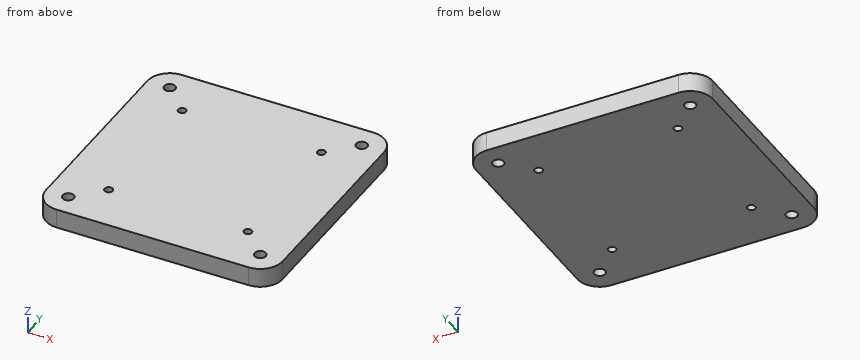
```python
from build123d import *

# Parameters (mm, degrees)
ESQUISSE1_W        = 74
ESQUISSE1_H        = 74
ESQUISSE1_R        = 1.75
ESQUISSE1_R_2      = 1.25
BOSS_EXTRU_1_DEPTH = 6
CONG_1_R           = 7


with BuildPart() as part:
    # Esquisse1 → Boss.-Extru.1 (new body)
    with BuildSketch(Plane.XY):
        Rectangle(ESQUISSE1_W, ESQUISSE1_H)
        with Locations((-30, 30)):
            Circle(ESQUISSE1_R, mode=Mode.SUBTRACT)
        with Locations((-21.75, 21.75)):
            Circle(ESQUISSE1_R_2, mode=Mode.SUBTRACT)
        with Locations((30, 30)):
            Circle(ESQUISSE1_R, mode=Mode.SUBTRACT)
        with Locations((21.75, 21.75)):
            Circle(ESQUISSE1_R_2, mode=Mode.SUBTRACT)
        with Locations((21.75, -21.75)):
            Circle(ESQUISSE1_R_2, mode=Mode.SUBTRACT)
        with Locations((-21.75, -21.75)):
            Circle(ESQUISSE1_R_2, mode=Mode.SUBTRACT)
        with Locations((-30, -30)):
            Circle(ESQUISSE1_R, mode=Mode.SUBTRACT)
        with Locations((30, -30)):
            Circle(ESQUISSE1_R, mode=Mode.SUBTRACT)
    extrude(amount=BOSS_EXTRU_1_DEPTH)

    # Congé1
    cong_1_edges = [part.edges().sort_by_distance(p)[0] for p in [
        (-37, 37, 3),
        (37, 37, 3),
        (37, -37, 3),
        (-37, -37, 3),
    ]]
    fillet(cong_1_edges, radius=CONG_1_R)


solid = part.part
```
Can you work these out from the model? Positions are in its coordinate system, mm. Round coordinates to 2 decimals unless told otherwise and drop trailing zeros. Loops run counter-clockwise (first coordinate to the right, second up) from the corner with the lowest first, then second, coordinate; pieces in that order, holes last.
Item 1: Suppose I cut it at A-A, the plane x = 21.75. Write out the boundary of the cut face in (y, z), then the cut area to 3 significant figures.
Item 2: Suppose I cut it at B-B, the plane z = 2.5. State how many separate pieces and enclosed holes the cut face has, then the cut area to 3 significant figures.
Item 3: Will this pin go through, and if not, where does the flat tip stop? pin 1 Ø5.5 at (x, y) = (30, 30) entering from +Z.
Item 4: Please list where these lines run through material, in increasing order: L1, parallel to Y at x = 21.75, z = 1.4; L2, parallel to Y at x = 30, z = 3.7; L3, parallel to X at y = 31.5, z = 1.1.
Reported:
1. outline: (-37, 0) - (-23, 0) - (-23, 6) - (-37, 6) - close; (-20.5, 0) - (20.5, 0) - (20.5, 6) - (-20.5, 6) - close; (23, 0) - (37, 0) - (37, 6) - (23, 6) - close
1. area: 414 mm2
2. separate pieces: 1
2. enclosed holes: 8
2. area: 5,380 mm2
3. pin 1: stops at z = 6
4. L1: y = -37 to -23, -20.5 to 20.5, 23 to 37
4. L2: y = -37 to -31.75, -28.25 to 28.25, 31.75 to 37
4. L3: x = -36.84 to -30.9, -29.1 to 29.1, 30.9 to 36.84
